Autodesk Inventor part; units mm, degrees
ref_plane "YZ Plane" through (0, 0, 0) normal (1, 0, 0) x (0, 1, 0)
ref_plane "XZ Plane" through (0, 0, 0) normal (0, 1, 0) x (-1, 0, 0)
ref_plane "XY Plane" through (0, 0, 0) normal (0, 0, 1) x (1, 0, 0)
sketch "Эскиз1" plane through (0, 0, 0) normal (0, 0, 1) x (1, 0, 0)
  circle A0 centre (0, 0) radius 20
  circle A1 centre (0, 0) radius 30
  dimension "d0" = 40
  dimension "d1" = 10
extrude "Выдавливание1" add sketch "Эскиз1" along normal blind 60
sketch "Эскиз2" plane through (0, 0, 0) normal (0, 0, -1) x (-1, 0, 0)
  circle A0 centre (0, 0) radius 30
extrude "Выдавливание2" add sketch "Эскиз2" along normal blind 10
sketch "Эскиз3" plane through (0, 0, -10) normal (0, 0, -1) x (-1, 0, 0)
  circle A0 centre (0, 0) radius 30
  line L0 (-29.5804, 5) -> (29.5804, 5)
  line L1 (29.5804, -5) -> (-29.5804, -5)
  line L2 (42, 0) -> (-42, 0)
  dimension "d7" = 10
extrude "Выдавливание3" add sketch "Эскиз3" along normal blind 20 contours L2 A0 L0 | A0 L1 L2
sketch "Эскиз4" plane through (-29.5804, 5, -10) normal (0, 1, 0) x (1, 0, 0)
  line L0 (59.1608, 0) -> (0, 0)
  line L1 (59.1608, 0) -> (59.1608, 20)
  line L2 (0, 20) -> (59.1608, 20)
  line L3 (0, 0) -> (0, 20)
  line L4 (59.1608, 0) -> (59.1608, 20)
  line L5 (0, 0) -> (59.1608, 0)
  line L6 (0, 0) -> (0, 20)
  line L7 (0, 20) -> (59.1608, 20)
  circle A0 centre (29.5804, 10) radius 5
  point P0 (29.5804, -10)
  dimension "d11" = 10
extrude "Выдавливание4" cut sketch "Эскиз4" along normal through all both and the other way through all contours A0
sketch "Эскиз5" plane through (-29.5804, -5, -10) normal (0, -1, 0) x (1, 0, 0)
  circle A0 centre (29.5804, -10) radius 5
  line L0 (59.1608, -20) -> (0, -20)
  line L1 (0, 0) -> (59.1608, 0)
  line L2 (0, 0) -> (0, -20)
  line L3 (16.199, -20) -> (0, 0)
  line L4 (0, 0) -> (-30.1779, 0)
  line L5 (-30.1779, 0) -> (-30.1779, -20)
  line L6 (-30.1779, -20) -> (16.199, -20)
  line L7 (42.9618, -20) -> (59.1608, 0)
  line L8 (85.3862, 0) -> (85.3862, -20)
  line L9 (85.3862, -20) -> (42.9618, -20)
  line L10 (85.3862, 0) -> (59.1608, 0)
  point P0 (29.5804, 10)
extrude "Выдавливание5" cut sketch "Эскиз5" against normal through all contours L0 L7 L10 L8 L9 | L0 L2 L3 | L6 L5 L4 L2
properties part number "стакан_v2" material "Сталь"
CAD build for the part. Positions are in the model's coordinates, mm. A direction names the side the tool comes from. Give positions to 0.01 mm unless a question says otherwise; leave off trailing zeros. Write each loop counter-clockwise with the first axis right and the second up, starting at its lowest first coordinate (ties: lowest second). Pieces come first, ordered by that corner, then holes. Notation, with made-up numbers: M 2,47.5 L 21,47.5 A11 ccw 21,59.5 Z; hole C 40.25,30.5 d1. An arc over 180 degrees is marked long. Return JSON: item names as keys, results as strings. Group by question number.
(1) Band-saw the part on D-D (x = 26). Give the cut face in (y, z), and give its area (3 significant figures).
(2) Flat gauge pins, fed straight in: pin 1 Ø1 at (x, y) = (10.5, 12) entering from -Z; pin 2 Ø9 at (x, z) = (0, -20) entering from +Y; pin 3 Ø22 at (x, z) = (-8, -22.5) entering from -Y; pin 4 Ø5 at (y, z) = (-1, -18) entering from +X. Where does each tip first touch, or does it go through?
(3) Drill centre lines: L1, parallel to Z at x = 0, y = -0.75; L2, parallel to Y at x = -0.5, z = 48.5; L3, parallel to Z at x = -13.5, y = 18. Where is each one in solid material? Low to high. Write a range as [from, to].
(4) Band-saw the part on B-B (z = -20). Give the cut face in (x, y).
(5) Band-saw the part on A-A (x = 0). Give the cut face in (y, z), and give its area (3 significant figures).
(6) 3-axis set-ups, long thin cutter, end or side, ignore diameter. For faces 4 (the face through (0, 15, -10)), 5 (the face through (0, 0, 0)), 6 (the face through (21.4, -0.1, -20.1)), 7 (the face through (0, -5, -13)): which of +Z, -Z, +X, -X, +Y, -Y reach the whole face in a straight line?
(7) Mould opens along X. For faces 1 (the face through (0, -15, -10)), 2 (the face through (-4.336, 19.524, 29.58)), 3 (the face through (-21.4, -0.1, -20.1)) say: pulls with the +X half, pulls with the -X half, needs draft (parallel to the pull), parting line crosses it, or undercut.
(8) Band-saw the part on C-C (y = 0). Give the cut face in (x, z).
Entries:
{
 "1": {"outline": "M -14.97,-10 L -5,-10 L -5,-14.42 L 5,-14.42 L 5,-10 L 14.97,-10 L 14.97,60 L -14.97,60 Z", "area": "2,140 mm^2"},
 "2": {"pin 1": "stops at z = -10", "pin 2": "passes through", "pin 3": "stops at y = -5", "pin 4": "stops at x = 25.13"},
 "3": {"L1": "z = [-30, -25], [-15, 0]", "L2": "y = [-30, -19.99], [19.99, 30]", "L3": "z = [-10, 60]"},
 "4": {"outline": "M -21.48,-5 L -5,-5 L -5,5 L -21.48,5 Z; M 5,-5 L 21.48,-5 L 21.48,5 L 5,5 Z"},
 "5": {"outline": "M -30,-10 L -5,-10 L -5,-15 L 5,-15 L 5,-10 L 30,-10 L 30,60 L 20,60 L 20,0 L -20,0 L -20,60 L -30,60 Z; M -5,-30 L 5,-30 L 5,-25 L -5,-25 Z", "area": "1,900 mm^2"},
 "6": {"face 4": "-Z, +X, -X, +Y", "face 5": "+Z", "face 6": "-Z, +X, +Y, -Y", "face 7": "-Z, +X, -X, -Y"},
 "7": {"face 1": "needs draft", "face 2": "undercut", "face 3": "pulls with the -X half"},
 "8": {"outline": "M -30,-10 L -29.58,-10 L -13.38,-30 L 13.38,-30 L 29.58,-10 L 30,-10 L 30,60 L 20,60 L 20,0 L -20,0 L -20,60 L -30,60 Z; hole C 0,-20 d10"}
}
